The figure shows three views and two pictorial views of one solid part (mm, origin at its lowest corner). Answer the questions. A direction names the side the tool comes from. Coordinates: 2 decimals unless noted, no trailing zeros. Order: outer loops, then holes, each group sorted by start corner. A loop starts at its lowest first (then second) coordinate and runs counter-clockwise, first axis right, second up. Notation, with made-up numbers: (48, 80) -> (53, 80) arc R22 ccw to (53, 101) -> close; hole circle Ø8 at (-33.75, 20). An arc over 180 degrees is marked (long way). Return JSON: item names as keys, results as strings.
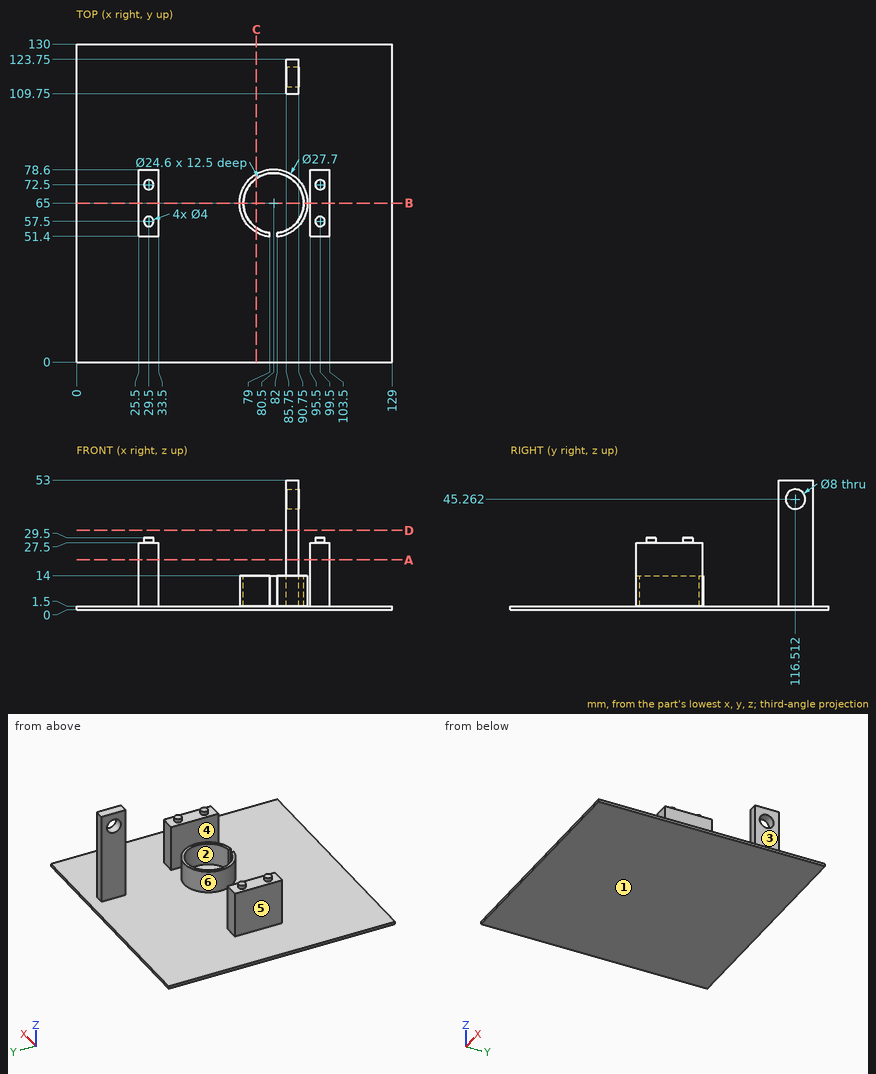
Item 1: The part is cut by section B-B on y = 65. Determine the outline of the cut face in (x, z).
Answer list:
{"outline": "(0, 0) -> (129, 0) -> (129, 1.5) -> (103.5, 1.5) -> (103.5, 27.5) -> (95.5, 27.5) -> (95.5, 1.5) -> (94.35, 1.5) -> (94.35, 14) -> (92.8, 14) -> (92.8, 1.5) -> (68.2, 1.5) -> (68.2, 14) -> (66.65, 14) -> (66.65, 1.5) -> (33.5, 1.5) -> (33.5, 27.5) -> (25.5, 27.5) -> (25.5, 1.5) -> (0, 1.5) -> close"}
Item 2: Determine the mould class of the marked faces 1 and 2 for opening direction Y: pulls with the +Y half, pulls with the -Y half, needs draft (parallel to the pull), parting line crosses it, or undercut.
Answer list:
{"face 1": "needs draft", "face 2": "undercut"}
Item 3: The part is cut by section A-A on z = 20.5. Determine the outline of the cut face in (x, y), plus the area to 3 significant figures.
Answer list:
{"outline": "(25.5, 51.4) -> (33.5, 51.4) -> (33.5, 78.6) -> (25.5, 78.6) -> close; (85.75, 109.75) -> (90.75, 109.75) -> (90.75, 123.75) -> (85.75, 123.75) -> close; (95.5, 51.4) -> (103.5, 51.4) -> (103.5, 78.6) -> (95.5, 78.6) -> close", "area": "505 mm2"}
Item 4: The part is cut by section C-C on x = 73.5. Determine the outline of the cut face in (y, z).
Answer list:
{"outline": "(0, 0) -> (130, 0) -> (130, 1.5) -> (76.95, 1.5) -> (76.95, 14) -> (75.11, 14) -> (75.11, 1.5) -> (54.89, 1.5) -> (54.89, 14) -> (53.05, 14) -> (53.05, 1.5) -> (0, 1.5) -> close"}
Item 5: Find the intervals of material crossed by probe 1 along X at (y, z) = (65, 4.5); probe 2 along X at (y, z) = (59, 4); probe 3 along Z at (x, y) = (41.5, 121.5), in increasing order.
Answer list:
{"probe 1": "25.5 to 33.5, 66.65 to 68.2, 92.8 to 94.35, 95.5 to 103.5", "probe 2": "25.5 to 33.5, 68.02 to 69.76, 91.24 to 92.98, 95.5 to 103.5", "probe 3": "0 to 1.5"}
Item 6: The part is cut by section D-D on z = 32.5. Determine the outline of the cut face in (x, y).
Answer list:
{"outline": "(85.75, 109.75) -> (90.75, 109.75) -> (90.75, 123.75) -> (85.75, 123.75) -> close"}
Item 7: Flat-ended cylindrical pins translate along their axes: pin 1 (13 mm diameter, centred on y = 67, z = 16, fed in from +X); pin 2 (2.5 mm diameter, centred on x = 31, z = 15.5, fed in from -Y); pin 3 (21 mm diameter, centred on y = 58.5, z = 16, fed in from -X); pin 4 (3 mm diameter, centred on x = 42.5, y = 38.5, fed in from -Z). Find the tip coordinate at first contact, or state that the pin passes through.
Answer list:
{"pin 1": "x = 103.5", "pin 2": "y = 51.4", "pin 3": "x = 25.5", "pin 4": "z = 0"}
Item 8: Which of the six approach directions +Z, -Z, +X, -X, +Y, -Y give full straight-line access (tool end or side, diameter ignored) to the marked faces 3, 4, 5 and 6?
Answer list:
{"face 3": "+Z, +X, +Y", "face 4": "+Z, +Y, -Y", "face 5": "+Z, -X, +Y, -Y", "face 6": "+Z"}
